Model file for the job. Use its own axes, mm. Face numbers are marked on the shaded views. A direction names the side the tool comes from. Round coordinates to 2 decimals unless told otherwise and drop trailing zeros. Loops run counter-clockwise (first coordinate to the right, second up) from the corner with the lowest first, then second, coordinate; pieces in that order, holes last. Notation, with made-up numbers: (71, -16.75) -> (118, -16.75) arc R22 ccw to (118, 22.25) -> close; hole circle Ø8 at (82, 80). An arc over 180 degrees is marked (long way). Use a Markdown table: item, result. Add a question column.
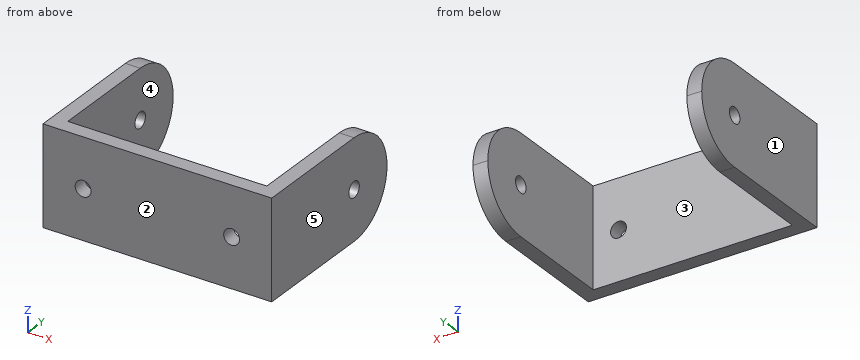
```python
from build123d import *

# Parameters (mm, degrees)
ESQUISSE1_W             = 40.2
ESQUISSE1_H             = 20
BOSS_EXTRU_1_DEPTH      = 3
ESQUISSE2_W             = 3
ESQUISSE2_H             = 20
BOSS_EXTRU_2_DEPTH      = 35
ENL_V_MAT_EXTRU_1_DEPTH = 71
ESQUISSE4_R             = 1.6
ENL_V_MAT_EXTRU_2_DEPTH = 71
ESQUISSE5_R             = 1.6
ENL_V_MAT_EXTRU_3_DEPTH = 71


with BuildPart() as part:
    # Esquisse1 → Boss.-Extru.1 (new body)
    with BuildSketch(Plane(origin=(0, 0, 0), x_dir=(1, 0, 0), z_dir=(0, 1, 0))):
        Rectangle(ESQUISSE1_W, ESQUISSE1_H)
    extrude(amount=BOSS_EXTRU_1_DEPTH)

    # Esquisse2 → Boss.-Extru.2 (add)
    with BuildSketch(Plane.XZ):
        with Locations((-21.6, 0)):
            Rectangle(ESQUISSE2_W, ESQUISSE2_H)
        with Locations((21.6, 0)):
            Rectangle(ESQUISSE2_W, ESQUISSE2_H)
    extrude(amount=-BOSS_EXTRU_2_DEPTH)

    # Esquisse3 → Enlèv. mat.-Extru.1 (cut)
    with BuildSketch(Plane(origin=(23.1, 0, 0), x_dir=(0, 0, -1), z_dir=(1, 0, 0))):
        with BuildLine():
            Line((-10, 35), (-10, 25))
            ThreePointArc((-10, 25), (-7.071067812, 32.071067812), (0, 35))
            Line((0, 35), (-10, 35))
        make_face()
        with BuildLine():
            Line((10, 35), (0, 35))
            ThreePointArc((0, 35), (7.071067812, 32.071067812), (10, 25))
            Line((10, 25), (10, 35))
        make_face()
    extrude(amount=-ENL_V_MAT_EXTRU_1_DEPTH, mode=Mode.SUBTRACT)

    # Esquisse4 → Enlèv. mat.-Extru.2 (cut)
    with BuildSketch(Plane(origin=(23.1, 0, 0), x_dir=(0, 0, -1), z_dir=(1, 0, 0))):
        with Locations((0, 25)):
            Circle(ESQUISSE4_R)
    extrude(amount=-ENL_V_MAT_EXTRU_2_DEPTH, mode=Mode.SUBTRACT)

    # Esquisse5 → Enlèv. mat.-Extru.3 (cut)
    with BuildSketch(Plane(origin=(0, 3, 0), x_dir=(1, 0, 0), z_dir=(0, 1, 0))):
        with Locations(Location((-15, 0, 0), (0, 0, 270))):
            Circle(ESQUISSE5_R)
        with Locations(Location((15, 0, 0), (0, 0, 270))):
            Circle(ESQUISSE5_R)
    extrude(amount=-ENL_V_MAT_EXTRU_3_DEPTH, mode=Mode.SUBTRACT)


solid = part.part
```
1) Cut at B-B on x = 15. Write the cut outline in (y, z), and give its area (3 significant figures).
2) Cut at D-D on z = -6. Write the cut outline in (x, y).
3) Tool access for the marked faces 4 and 5: list every direction of +Z, -Z, +X, -X, +Y, -Y with a clear straight run to the whole face (end or side of a thin tool).
4) Cut at C-C on z = 1. Write the cut outline in (x, y), and give its area (3 significant figures).
5) Wall check: probe 1 along X at (y, z) = (1.45, 0); probe 2 along X at (y, z) = (10.5, 1); probe 3 along Y at (x, z) = (22.45, 0). Give the ranges that are in metal, low to high. Write a range as from..to.
6) Cut at A-A on y = 21.5. Write the cut outline in (x, z).
7) Pin check, flat tip, straight feed: pin 1 Ø6 at (x, z) = (-3, 4) entering from +Y. Stop position of the tip, or through.
8) Pull direction X, two halves, no side cores. Call the marked faces 1, 2 and 3: +X half, -X half, draft (parallel to the pull), parting line (faces both ways), or undercut.
Established:
| question | item | result |
|---|---|---|
| 1 | outline | (0, -10) -> (3, -10) -> (3, -1.6) -> (0, -1.6) -> close; (0, 1.6) -> (3, 1.6) -> (3, 10) -> (0, 10) -> close |
| 1 | area | 50.4 mm^2 |
| 2 | outline | (-23.1, 0) -> (23.1, 0) -> (23.1, 33) -> (20.1, 33) -> (20.1, 3) -> (-20.1, 3) -> (-20.1, 33) -> (-23.1, 33) -> close |
| 3 | face 4 | +Z, -Z, +Y |
| 3 | face 5 | +Z, -Z, +X, +Y, -Y |
| 4 | outline | (-23.1, 0) -> (-16.25, 0) -> (-16.25, 3) -> (-20.1, 3) -> (-20.1, 23.75) -> (-23.1, 23.75) -> close; (-23.1, 26.25) -> (-20.1, 26.25) -> (-20.1, 34.95) -> (-23.1, 34.95) -> close; (-13.75, 0) -> (13.75, 0) -> (13.75, 3) -> (-13.75, 3) -> close; (16.25, 0) -> (23.1, 0) -> (23.1, 23.75) -> (20.1, 23.75) -> (20.1, 3) -> (16.25, 3) -> close; (20.1, 26.25) -> (23.1, 26.25) -> (23.1, 34.95) -> (20.1, 34.95) -> close |
| 4 | area | 300 mm^2 |
| 5 | probe 1 | x = -23.1..-16.6, -13.4..13.4, 16.6..23.1 |
| 5 | probe 2 | x = -23.1..-20.1, 20.1..23.1 |
| 5 | probe 3 | y = 0..23.4, 26.6..35 |
| 6 | outline | (-23.1, -10) -> (-20.1, -10) -> (-20.1, 10) -> (-23.1, 10) -> close; (20.1, -10) -> (23.1, -10) -> (23.1, 10) -> (20.1, 10) -> close |
| 7 | pin 1 | stops at y = 3 |
| 8 | face 1 | -X half |
| 8 | face 2 | draft |
| 8 | face 3 | undercut |
